```python
from build123d import *

# Parameters (mm, degrees)
SKETCH1_W           = 171
SKETCH1_H           = 70
SKETCH1_R           = 2.25
BOSS_EXTRUDE1_DEPTH = 5
SKETCH2_W           = 171
SKETCH2_H           = 65
SKETCH2_R           = 2.25
BOSS_EXTRUDE2_DEPTH = 3
CHAMFER1_SIZE       = 8
CHAMFER3_SIZE       = 3
SKETCH3_W           = 7.071067812
SKETCH3_H           = 2.6
CUT_EXTRUDE1_DEPTH  = 199.002168661
SKETCH4_R           = 29
SKETCH4_R_2         = 1.75
SKETCH4_W           = 48
SKETCH4_H           = 29
CUT_EXTRUDE2_DEPTH  = 185.945938047


with BuildPart() as part:
    # Sketch1 → Boss-Extrude1 (new body)
    with BuildSketch(Plane.XY):
        with Locations((85.5, 35)):
            Rectangle(SKETCH1_W, SKETCH1_H)
        with Locations((15, 9)):
            Circle(SKETCH1_R, mode=Mode.SUBTRACT)
        with Locations(Location((156, 9, 0), (0, 0, 180))):
            Circle(SKETCH1_R, mode=Mode.SUBTRACT)
        with Locations((15, 58)):
            Circle(SKETCH1_R, mode=Mode.SUBTRACT)
        with Locations(Location((156, 58, 0), (0, 0, 180))):
            Circle(SKETCH1_R, mode=Mode.SUBTRACT)
    extrude(amount=-BOSS_EXTRUDE1_DEPTH)

    # Sketch2 → Boss-Extrude2 (add)
    with BuildSketch(Plane(origin=(0, 0, -5), x_dir=(-1, 0, 0), z_dir=(0, 0, -1))):
        with Locations((-85.5, 37.5)):
            Rectangle(SKETCH2_W, SKETCH2_H)
        with Locations(Location((-15, 9, 0), (0, 0, 180))):
            Circle(SKETCH2_R, mode=Mode.SUBTRACT)
        with Locations((-156, 9)):
            Circle(SKETCH2_R, mode=Mode.SUBTRACT)
        with Locations(Location((-15, 58, 0), (0, 0, 180))):
            Circle(SKETCH2_R, mode=Mode.SUBTRACT)
        with Locations((-156, 58)):
            Circle(SKETCH2_R, mode=Mode.SUBTRACT)
    extrude(amount=BOSS_EXTRUDE2_DEPTH)

    # Chamfer1
    # the kernel refuses this chamfer: 8 mm, written as the material it takes off along each edge
    with BuildSketch(Plane(origin=(171, -15.573463904, -8), x_dir=(-0.9996219169112968, 0, -0.027495876610586296), z_dir=(0, 1, 0)), Plane(origin=(0, 90.573463904, -8), x_dir=(0.9996219169112968, 0, -0.027495876610586275), z_dir=(0, -1, 0))) as chamfer1_piece_1:
        Polygon((CHAMFER1_SIZE * 0.999621916911, CHAMFER1_SIZE * 0.0274958766106), (-CHAMFER1_SIZE * 0.0274958766106, CHAMFER1_SIZE * 0.999621916911), (0, 0), align=None)
    extrude(amount=106.146927807, mode=Mode.SUBTRACT)

    # Chamfer3
    chamfer3_edges = [part.edges().sort_by_distance(p)[0] for p in [
        (85.5, 70, -8),
    ]]
    chamfer(chamfer3_edges, length=CHAMFER3_SIZE)

    # Sketch3 → Cut-Extrude1 (cut, through all, along a direction that is not the sketch's normal)
    with BuildSketch(Plane(origin=(85.5, 0, -85.5), x_dir=(-0.7071067811865452, 0, -0.7071067811865498), z_dir=(0.7071067811865498, 0, -0.7071067811865452))):
        with Locations((-117.379725677, 1.3)):
            Rectangle(SKETCH3_W, SKETCH3_H)
    extrude(amount=-CUT_EXTRUDE1_DEPTH, dir=(1, 0, 0), mode=Mode.SUBTRACT)

    # Sketch4 → Cut-Extrude2 (cut, through all)
    with BuildSketch(Plane.XY):
        with Locations((58, 36.3)):
            Circle(SKETCH4_R)
        with Locations((33, 60.3)):
            Circle(SKETCH4_R_2)
        with Locations((83, 60.3)):
            Circle(SKETCH4_R_2)
        with Locations((83, 10.3)):
            Circle(SKETCH4_R_2)
        with Locations((33, 10.3)):
            Circle(SKETCH4_R_2)
        with Locations((117, 60.5)):
            Circle(SKETCH4_R_2)
        with Locations((117, 20.5)):
            Circle(SKETCH4_R_2)
        with Locations((117, 40.5)):
            Rectangle(SKETCH4_W, SKETCH4_H)
    extrude(amount=-CUT_EXTRUDE2_DEPTH, mode=Mode.SUBTRACT)


solid = part.part
```
CAD build for the part. Positions are in the model's coordinates, mm. A direction names the side the tool comes from. Coordinates: 2 decimals unless noted, no trailing zeros. Order: outer loops, then holes, each group sorted by start corner. A loop starts at its lowest first (then second) coordinate and runs counter-clockwise, first axis right, second up.
(1) Saw through at C-C, the plane z = -2.5. Count the separate pieces of the cut face and the enclosed holes in it, and give its area (3 significant figures).
Solution:
separate pieces: 1
enclosed holes: 12
area: 7,030 mm2
(2) Saw through at A-A, the plane x = 117. Write the cut outline in (y, z), and give its area (4 significant figures).
Solution:
outline: (2.6, -5) - (5, -5) - (5, -8) - (18.75, -8) - (18.75, 0) - (2.6, 0) - close; (22.25, -8) - (26, -8) - (26, 0) - (22.25, 0) - close; (55, -8) - (58.75, -8) - (58.75, 0) - (55, 0) - close; (62.25, -8) - (67, -8) - (70, -5) - (70, 0) - (62.25, 0) - close
area: 239.5 mm2
(3) Pin check, flat tips, straight feed: pin 1 Ø1 at (x, z) = (139, -7) entering from +Y; pin 2 Ø2.5 at (x, y) = (110, 3.5) entering from -Z; pin 3 Ø3.5 at (x, y) = (156, 9) entering from +Z; pin 4 Ø1 at (y, z) = (59.5, -1.5) entering from +X. Stop position of each tip, or through.
Solution:
pin 1: stops at y = 68.5
pin 2: stops at z = -5
pin 3: passes through
pin 4: stops at x = 170
(4) Which spindle directions (+Z, -Z, +X, -X, +Y, -Y) get a long thin tool onto all of the face, cutting with end or side? Do faces 5 (the face through (83, 2.6, -3)), 6 (the face through (141, 40, -4)). Say none if no direction does.
Solution:
face 5: +Z, -Z, +X, -X, -Y
face 6: +Z, -Z
(5) Saw through at B-B, the plane y = 31.5. Write the cut outline in (x, z).
Solution:
outline: (0, 0) - (8, -8) - (29.4, -8) - (29.4, 0) - close; (86.6, -8) - (93, -8) - (93, 0) - (86.6, 0) - close; (141, -8) - (163, -8) - (171, 0) - (141, 0) - close
(6) Saw through at D-D, the plane x = 15. Write the cut outline in (y, z), and give its area (4 significant figures).
Solution:
outline: (2.6, -5) - (5, -5) - (5, -8) - (6.75, -8) - (6.75, 0) - (2.6, 0) - close; (11.25, -8) - (55.75, -8) - (55.75, 0) - (11.25, 0) - close; (60.25, -8) - (67, -8) - (70, -5) - (70, 0) - (60.25, 0) - close
area: 455.5 mm2
(7) Drill centre lines: L1, parallel to Y at x = 121.5, z = -1.5; L2, parallel to Y at x = 156, z = -6.65; L3, parallel to X at y = 58, z = -7.05. Where is each one in solid material? Low to high.
Solution:
L1: y = 2.6 to 26, 55 to 70
L2: y = 5 to 6.75, 11.25 to 55.75, 60.25 to 68.35
L3: x = 7.05 to 12.75, 17.25 to 38.76, 77.24 to 153.75, 158.25 to 163.95
(8) Mould opens along X. For faces 1 (the face through (87, 30, -8)), 2 (the face through (4, 37, -4)), 3 (the face through (31.71, 61.48, -3.94)), 4 (the face through (167, 36, -4)) say: released by +X, released by -X, zero draft, split by the parting line, or undercut.
Solution:
face 1: zero draft
face 2: released by -X
face 3: undercut
face 4: released by +X
